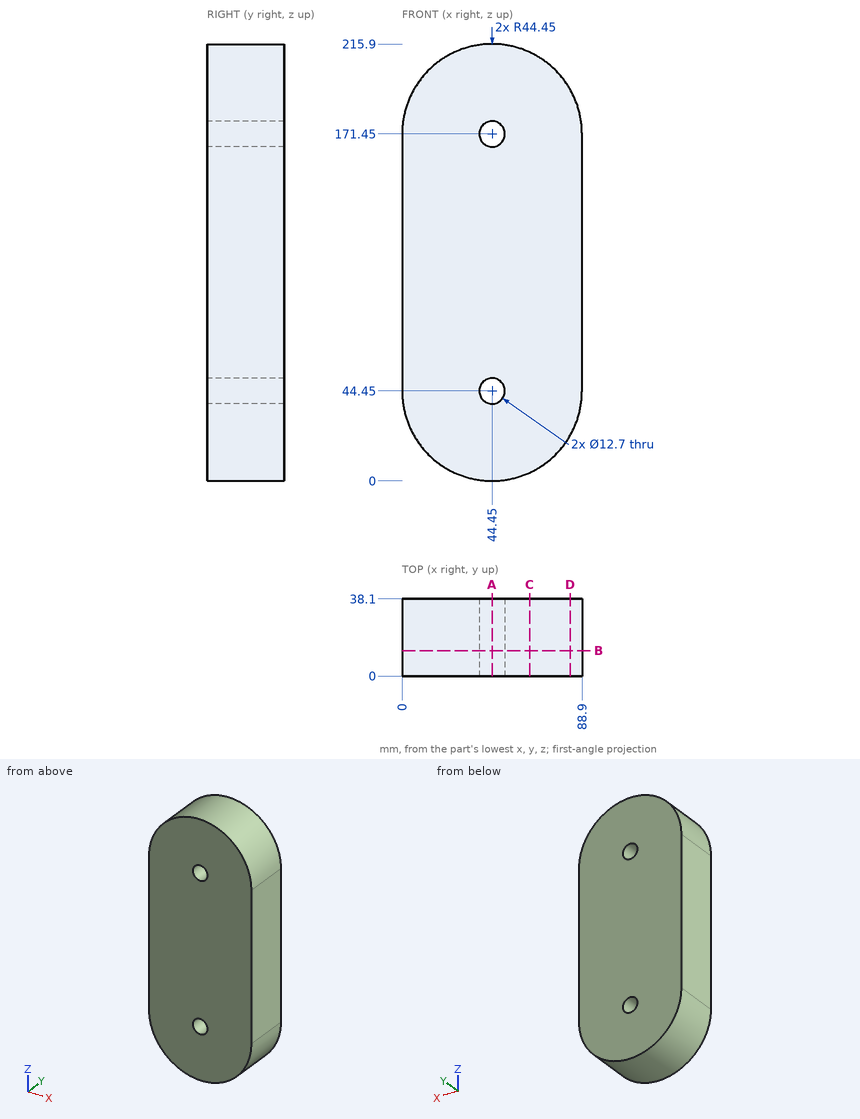
Design review of the part shown in the three views and the two pictorial views. Dimensions are in mm from the part's minimum x, y and z. Give positions to 0.01 mm unless a question says otherwise; leave off trailing zeros. Loops run counter-clockwise (first coordinate to the right, second up) from the corner with the lowest first, then second, coordinate; pieces in that order, holes last. Notation, with made-up numbers: (68.5, 43.5) -> (90.5, 43.5) arc R28 ccw to (90.5, 78.5) -> close; hole circle Ø11 at (55.25, -25). An arc over 180 degrees is marked (long way). Answer as a JSON object with one key per item and string values. Group by question number.
Q1. Take a section at C-C (x = 63). Write out the cut boundary in (y, z).
Q2. Wall thickness on line 1 along Z through (x, y) = (44.45, 17); line 2 along X through (y, z) = (24.5, 44.45); line 3 along Z through (x, y) = (43.5, 16.5): over which ranges is each line inside the solid? List them lowest first.
Q3. Take a section at D-D (x = 83). Write out the cut boundary in (y, z), plus the area to 3 significant figures.
Q4. Insertion check: pin 1 (5 mm diameter, centred on y = 23, z = 22, fed in from +X); pin 2 (1.5 mm diameter, centred on x = 54.5, y = 30.5, fed in from -Z); pin 3 (4 mm diameter, centred on x = 30, y = 24, fed in from -Z). Each pin has a flat end and moves straight along its axis. Give the tip position at first contact, or say it passes through.
Q5. Take a section at B-B (y = 12.5). Write out the cut boundary in (x, z).
Q6. Take a section at A-A (x = 44.45). Write out the cut boundary in (y, z).
Answer below:
{
 "1": {"outline": "(0, 4.06) -> (38.1, 4.06) -> (38.1, 211.84) -> (0, 211.84) -> close"},
 "2": {"line 1": "z = 0 to 38.1, 50.8 to 165.1, 177.8 to 215.9", "line 2": "x = 0 to 38.1, 50.8 to 88.9", "line 3": "z = 0.01 to 38.17, 50.73 to 165.17, 177.73 to 215.89"},
 "3": {"outline": "(0, 22.32) -> (38.1, 22.32) -> (38.1, 193.58) -> (0, 193.58) -> close", "area": "6,520 mm2"},
 "4": {"pin 1": "stops at x = 84.17", "pin 2": "stops at z = 0.98", "pin 3": "stops at z = 1.78"},
 "5": {"outline": "(0, 44.45) arc R44.45 ccw to (88.9, 44.45) -> (88.9, 171.45) arc R44.45 ccw to (0, 171.45) -> close; hole circle Ø12.7 at (44.45, 44.45); hole circle Ø12.7 at (44.45, 171.45)"},
 "6": {"outline": "(0, 0) -> (38.1, 0) -> (38.1, 38.1) -> (0, 38.1) -> close; (0, 50.8) -> (38.1, 50.8) -> (38.1, 165.1) -> (0, 165.1) -> close; (0, 177.8) -> (38.1, 177.8) -> (38.1, 215.9) -> (0, 215.9) -> close"}
}
